Could you check a few things on this model? Use its own coordinates, in mm. Face numbers are marked on the shaded views. A direction names the side the tool comes from. Give positions to 0.01 mm unless a question says otherwise; leave off trailing zeros. Loops run counter-clockwise (first coordinate to the right, second up) from the corner with the lowest first, then second, coordinate; pieces in that order, holes last. Notation, with made-up numbers: M 77.5,-15 L 90.5,-15 A10 cw 90.5,1 Z; hole C 74,-17 d8. An arc over 180 degrees is marked long. Use a Markdown table: item, result. Add a question column.
1) Suppose I cut it at C-C on z = -14. Count the separate pieces of the cut face and the enclosed holes in it, and give its area (3 significant figures).
2) If I drill on line 1 along Y through (x, z) = (0, 2.5); line 2 along Y through (x, z) = (-28, -2) (3 decimals); line 3 along X through (y, z) = (18, 6), over which ranges is the centre line in solid material (lowest first)? Write a range as [from, to].
3) Will these pins go through, and if not, where does the flat tip stop? pin 1 Ø8 at (x, y) = (27.93, -38.45) entering from +Z; pin 2 Ø10 at (y, z) = (-27.5, -5) entering from +X; pin 3 Ø8 at (x, z) = (-10.5, 14.5) entering from +Y; pin 4 Ø6 at (x, z) = (-42, 10.5) entering from -Y.
4) Suppose I cut it at B-B on x = 30.5. List the corners of the cut face in (y, z) for me (3 decimals), and give its area (3 significant figures).
5) Suppose I cut it at A-A on y = -4. List the corners of the cut face in (x, z) for me (3 decimals), and give its area (3 significant figures).
6) We'd pull the mould along Y, two halves only. Please class the marked faces 1, 2, 3 and 4: +Y half, -Y half, draft (parallel to the pull), parting line (faces both ways), or undercut.
7) Which directions (+Z, -Z, +X, -X, +Y, -Y) give clear straight access to the entire face, cutting with the end or side of a thin tool? Please do the marked faces 5 and 6.
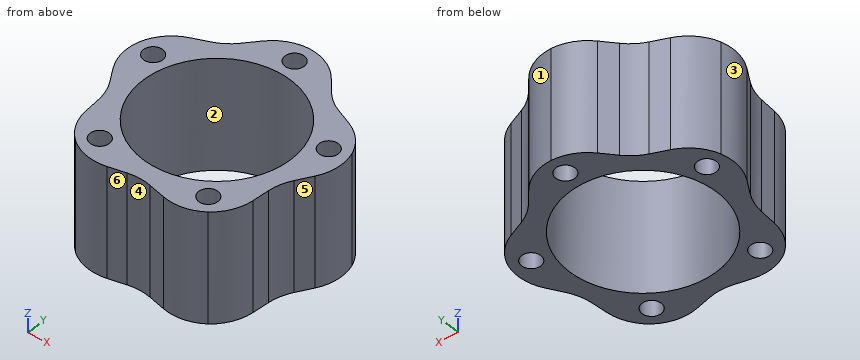
```python
from build123d import *

# Parameters (mm, degrees)
SKETCH1_R                        = 57.15
SKETCH1_R_2                      = 38.1
BOSS_EXTRUDE1_DEPTH              = 28.575
F_25_64_0_39063_DIAMETER_HOLE2_D = 9.921875
CIRPATTERN2_COUNT                = 5
CUT_EXTRUDE2_DEPTH               = 99.986703653
FILLET1_R                        = 23.8125
FILLET2_R                        = 25.4
CIRPATTERN1_START                = -28.575
CIRPATTERN1_DEPTH                = 57.15


# Read off the part's stored shape, not the designer's step: CirPattern1
with BuildPart() as part:
    # Sketch1 → Boss-Extrude1 (new, symmetric)
    with BuildSketch(Plane.XY):
        Circle(SKETCH1_R)
        Circle(SKETCH1_R_2, mode=Mode.SUBTRACT)
    extrude(amount=BOSS_EXTRUDE1_DEPTH, both=True)

    # 25/64 (0.39063) Diameter Hole2 (through all)
    with Locations(Plane.XY.offset(28.575)):
        with Locations((0, 47.5234)):
            f_25_64_0_39063_diameter_hole2 = Hole(F_25_64_0_39063_DIAMETER_HOLE2_D / 2)

    # CirPattern2: 25/64 (0.39063) Diameter Hole2 ×5 about axis
    cirpattern2_axis = Axis((0, 0, 0), (0, 0, 1))
    for i in range(1, CIRPATTERN2_COUNT):
        add(f_25_64_0_39063_diameter_hole2.rotate(cirpattern2_axis, i * 360 / CIRPATTERN2_COUNT), mode=Mode.SUBTRACT)

    # Sketch5 → Cut-Extrude2 (cut, through all)
    with BuildSketch(Plane.XY.offset(28.575)):
        Polygon((0, -46.54915497), (88.85993875, -67.46875), (-88.85993875, -67.46875), align=None)
    extrude(amount=-CUT_EXTRUDE2_DEPTH, mode=Mode.SUBTRACT)

    # Fillet1
    fillet1_edges = [part.edges().sort_by_distance(p)[0] for p in [
        (23.519318129, -52.086122669, 0),
        (-23.519318129, -52.086122669, 0),
    ]]
    fillet(fillet1_edges, radius=FILLET1_R)

    # Fillet2
    fillet2_edges = [part.edges().sort_by_distance(p)[0] for p in [
        (0, -46.54915497, 0),
    ]]
    fillet(fillet2_edges, radius=FILLET2_R)

    # CirPattern1 outline → CirPattern1 (cut)
    with BuildSketch(Plane.XY.offset(CIRPATTERN1_START)):
        with BuildLine():
            ThreePointArc((-43.775443864, -20.343642549), (-44.931279172, -14.59905758), (-47.372771091, -9.272207766))
            Line((-47.372771091, -9.272207766), (-51.967174053, -1.7001118))
            ThreePointArc((-51.967174053, -1.7001118), (-55.202463072, 7.429620219), (-54.5340897, 17.092558633))
            ThreePointArc((-54.5340897, 17.092558633), (-54.352879906, -17.660321229), (-34.072251451, -45.882504084))
            ThreePointArc((-34.072251451, -45.882504084), (-40.292709561, -38.457882702), (-43.041627602, -29.170119173))
            Line((-43.041627602, -29.170119173), (-43.775443864, -20.343642549))
        make_face()
        with BuildLine():
            ThreePointArc((34.072251451, -45.882504084), (54.534089699, -17.092558633), (54.165759228, 18.226163261))
            ThreePointArc((54.165759228, 18.226163261), (55.264246489, 8.008560011), (51.954827504, -1.72046031))
            Line((51.954827504, -1.72046031), (47.372771091, -9.272207766))
            ThreePointArc((47.372771091, -9.272207766), (44.931279172, -14.59905758), (43.775443864, -20.343642549))
            Line((43.775443864, -20.343642549), (43.041627602, -29.170119173))
            ThreePointArc((43.041627602, -29.170119173), (40.292709561, -38.457882702), (34.072251451, -45.882504084))
        make_face()
        with BuildLine():
            ThreePointArc((54.165759228, 18.226163261), (33.107949758, 46.583110274), (-0.595971221, 57.146892464))
            ThreePointArc((-0.595971221, 57.146892464), (9.460998162, 55.034202885), (17.691179628, 48.880325777))
            Line((17.691179628, 48.880325777), (23.457384954, 42.188912866))
            ThreePointArc((23.457384954, 42.188912866), (27.769057686, 38.220828948), (32.875309902, 35.346389866))
            Line((32.875309902, 35.346389866), (41.043026315, 31.92095785))
            ThreePointArc((41.043026315, 31.92095785), (49.026751951, 26.436504665), (54.165759228, 18.226163261))
        make_face()
        with BuildLine():
            ThreePointArc((-0.595971221, 57.146892464), (-34.072251451, 45.882504084), (-54.5340897, 17.092558633))
            ThreePointArc((-54.5340897, 17.092558633), (-49.417028058, 26.004447915), (-41.021077193, 31.930163021))
            Line((-41.021077193, 31.930163021), (-32.875309902, 35.346389866))
            ThreePointArc((-32.875309902, 35.346389866), (-27.769057686, 38.220828948), (-23.457384954, 42.188912866))
            Line((-23.457384954, 42.188912866), (-17.675642338, 48.898356078))
            ThreePointArc((-17.675642338, 48.898356078), (-9.992510498, 54.796541129), (-0.595971221, 57.146892464))
        make_face()
    extrude(amount=CIRPATTERN1_DEPTH, mode=Mode.SUBTRACT)


solid = part.part
```
Answer block:
| question | item | result |
|---|---|---|
| 1 | separate pieces | 1 |
| 1 | enclosed holes | 6 |
| 1 | area | 3,750 mm^2 |
| 2 | line 1 | y = [-47.24, -38.1], [38.1, 42.56], [52.48, 57.15] |
| 2 | line 2 | y = [-49.148, -43.408], [-33.487, -25.838], [25.838, 38.055] |
| 2 | line 3 | x = [-54.23, -48.89], [-41.51, -33.58], [33.58, 41.51], [48.89, 54.24] |
| 3 | pin 1 | passes through |
| 3 | pin 2 | stops at x = 43.6 |
| 3 | pin 3 | stops at y = 56.16 |
| 3 | pin 4 | stops at y = -40.59 |
| 4 | outline | M -48.076,-28.575 L -42.693,-28.575 L -42.693,28.575 L -48.076,28.575 Z; M -34.202,-28.575 L -22.833,-28.575 L -22.833,28.575 L -34.202,28.575 Z; M 22.833,-28.575 L 36.491,-28.575 L 36.491,28.575 L 22.833,28.575 Z |
| 4 | area | 1,740 mm^2 |
| 5 | outline | M -50.572,-28.575 L -37.889,-28.575 L -37.889,28.575 L -50.572,28.575 Z; M 37.889,-28.575 L 50.572,-28.575 L 50.572,28.575 L 37.889,28.575 Z |
| 5 | area | 1,450 mm^2 |
| 6 | face 1 | +Y half |
| 6 | face 2 | undercut |
| 6 | face 3 | parting line |
| 6 | face 4 | -Y half |
| 7 | face 5 | +Z, -Z, +X, -Y |
| 7 | face 6 | +Z, -Z, -Y |
